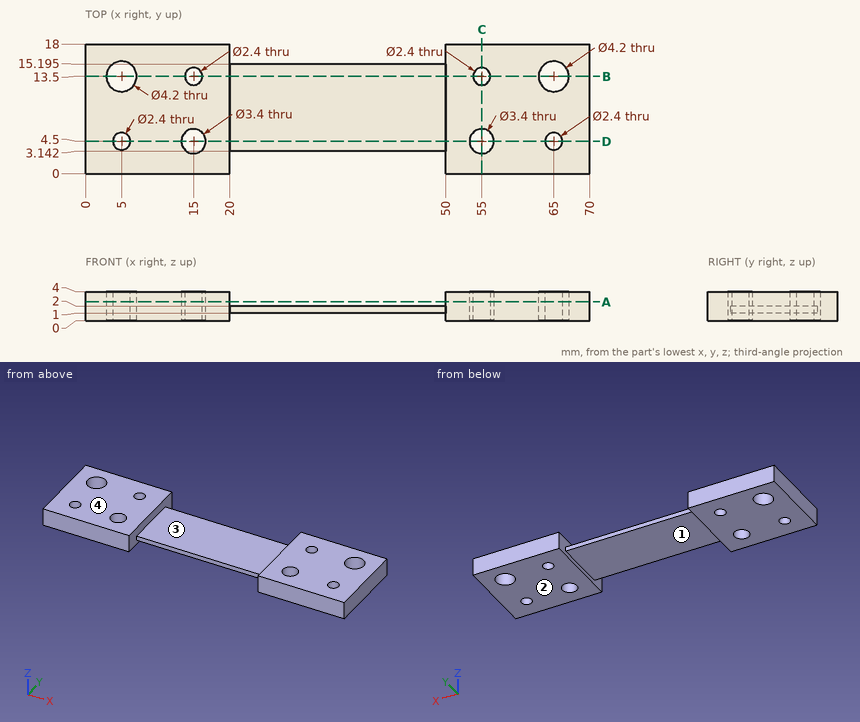
Could you check a few things on this drawing? It's one solid part, dimensions in mm from its lowest x, y, z. A direction names the side the tool comes from. Coordinates: 2 decimals unless noted, no trailing zeros. Write each loop counter-clockwise with the first axis right and the second up, starting at its lowest first coordinate (ties: lowest second). Pieces come first, ordered by that corner, then holes. Notation, with made-up numbers: (-25, 7.25) - (7, 7.25) arc R26 ccw to (7, 22.25) - close; hole circle Ø3 at (38, 22). An arc over 180 degrees is marked (long way). Put each result on its own line as item: value. Start each with the question number.
Q1. I'm going to push flat-ended pins straight in: P1, Ø1.1, axis at x = 36.5, z = 1.5, coming from the -Y side; P2, Ø3, axis at x = 39, y = 16, coming from the +Z side; P3, Ø8, axis at x = 36, y = 13.5, coming from the -Z side; P4, Ø2.5, axis at x = 5, y = 13.5, coming from the -Z side. Where does each tip first touch, or does it pass through?
Q2. Which directions (+Z, -Z, +X, -X, +Y, -Y) give clear straight access to the entire face, cutting with the end or side of a thin tool? Please do the marked faces 3 and 4.
Q3. Thinking about a two-plate mould opening in X: for the marked faces 1 and 2, which applies, pulls with the +X half, pulls with the -X half, needs draft (parallel to the pull), parting line crosses it, or undercut?
Q4. I want a section at B-B on y = 13.5. Write out the boundary of the cut face in (x, z), plus the area to 3 significant figures.
Q5. I want a section at D-D on y = 4.5. Write out the boundary of the cut face in (x, z).
Q6. I want a section at A-A on z = 2.6. Count the separate pieces of the cut face and the enclosed holes in it, plus the area to 3 significant figures.
Q7. I want a section at C-C on x = 55. Write out the boundary of the cut face in (y, z), plus the area to 3 significant figures.
Q8. Please list where these lines run through material, in increasing order: L1, parallel to Y at x = 65, z = 1.2; L2, parallel to Y at x = 15, z = 2.6; L3, parallel to X at y = 8.25, z = 2.75.
Checks:
1. P1: y = 3.14
1. P2: z = 2
1. P3: z = 1
1. P4: through
2. face 3: +Z, +Y, -Y
2. face 4: +Z, +X, -X, +Y, -Y
3. face 1: undercut
3. face 2: needs draft
4. outline: (0, 0) - (2.9, 0) - (2.9, 4) - (0, 4) - close; (7.1, 0) - (13.8, 0) - (13.8, 4) - (7.1, 4) - close; (16.2, 0) - (20, 0) - (20, 1) - (50, 1) - (50, 0) - (53.8, 0) - (53.8, 4) - (50, 4) - (50, 2) - (20, 2) - (20, 4) - (16.2, 4) - close; (56.2, 0) - (62.9, 0) - (62.9, 4) - (56.2, 4) - close; (67.1, 0) - (70, 0) - (70, 4) - (67.1, 4) - close
4. area: 137 mm²
5. outline: (0, 0) - (3.8, 0) - (3.8, 4) - (0, 4) - close; (6.2, 0) - (13.3, 0) - (13.3, 4) - (6.2, 4) - close; (16.7, 0) - (20, 0) - (20, 1) - (50, 1) - (50, 0) - (53.3, 0) - (53.3, 4) - (50, 4) - (50, 2) - (20, 2) - (20, 4) - (16.7, 4) - close; (56.7, 0) - (63.8, 0) - (63.8, 4) - (56.7, 4) - close; (66.2, 0) - (70, 0) - (70, 4) - (66.2, 4) - close
6. separate pieces: 2
6. enclosed holes: 8
6. area: 656 mm²
7. outline: (0, 0) - (2.8, 0) - (2.8, 4) - (0, 4) - close; (6.2, 0) - (12.3, 0) - (12.3, 4) - (6.2, 4) - close; (14.7, 0) - (18, 0) - (18, 4) - (14.7, 4) - close
7. area: 48.8 mm²
8. L1: 0 to 3.3, 5.7 to 11.4, 15.6 to 18
8. L2: 0 to 2.8, 6.2 to 12.3, 14.7 to 18
8. L3: 0 to 20, 50 to 70
